from build123d import *

# Parameters (mm, degrees)
SKIZZE1_R                       = 18.5
LINEAR_AUSTRAGEN1_DEPTH         = 1.8
SKIZZE2_R                       = 23.4
SKIZZE2_R_2                     = 18.5
LINEAR_AUSTRAGEN2_DEPTH         = 1
SKIZZE3_R                       = 1
SCHNITT_LINEAR_AUSTRAGEN1_DEPTH = 34.832857329
CHAMFER1_SIZE                   = 1.4
SKETCH1_R                       = 5
CUT_EXTRUDE1_DEPTH              = 10


with BuildPart() as part:
    # Skizze1 → Linear austragen1 (new body)
    with BuildSketch(Plane.XY):
        with BuildLine():
            ThreePointArc((-22.806936421, 5.234849671), (-23.4, 0), (-22.806936421, -5.234849671))
            ThreePointArc((-22.806936421, -5.234849671), (-22.254722481, -7.230997668), (-21.528166589, -9.170498531))
            ThreePointArc((-21.528166589, -9.170498531), (-21.322328126, -10.083900652), (-21.453393631, -11.010990043))
            ThreePointArc((-21.453393631, -11.010990043), (-21.560643818, -12.043510102), (-21.221833257, -13.024737741))
            ThreePointArc((-21.221833257, -13.024737741), (-20.14452316, -14.635852782), (-18.94516883, -16.158297497))
            ThreePointArc((-18.94516883, -16.158297497), (-18.116664111, -16.783741505), (-17.10153705, -17.000806761))
            ThreePointArc((-17.10153705, -17.000806761), (-16.179321175, -17.162642436), (-15.37423172, -17.640663225))
            ThreePointArc((-15.37423172, -17.640663225), (-13.754174904, -18.930997668), (-12.026368835, -20.073027989))
            ThreePointArc((-12.026368835, -20.073027989), (-11.322957725, -20.690997014), (-10.884062474, -21.518066457))
            ThreePointArc((-10.884062474, -21.518066457), (-10.363929634, -22.416432811), (-9.513074997, -23.011114795))
            ThreePointArc((-9.513074997, -23.011114795), (-7.69452316, -23.681307256), (-5.829354574, -24.208028116))
            ThreePointArc((-5.829354574, -24.208028116), (-4.791453413, -24.227040092), (-3.842610612, -23.805972857))
            ThreePointArc((-3.842610612, -23.805972857), (-3.001397674, -23.394835778), (-2.069093052, -23.308343012))
            ThreePointArc((-2.069093052, -23.308343012), (0, -23.4), (2.069093052, -23.308343012))
            ThreePointArc((2.069093052, -23.308343012), (3.001397674, -23.394835778), (3.842610612, -23.805972857))
            ThreePointArc((3.842610612, -23.805972857), (4.791453413, -24.227040092), (5.829354574, -24.208028116))
            ThreePointArc((5.829354574, -24.208028116), (7.69452316, -23.681307256), (9.513074997, -23.011114795))
            ThreePointArc((9.513074997, -23.011114795), (10.363929634, -22.416432811), (10.884062474, -21.518066457))
            ThreePointArc((10.884062474, -21.518066457), (11.322957725, -20.690997014), (12.026368835, -20.073027989))
            ThreePointArc((12.026368835, -20.073027989), (13.754174904, -18.930997668), (15.37423172, -17.640663225))
            ThreePointArc((15.37423172, -17.640663225), (16.179321175, -17.162642436), (17.10153705, -17.000806761))
            ThreePointArc((17.10153705, -17.000806761), (18.116664111, -16.783741505), (18.94516883, -16.158297497))
            ThreePointArc((18.94516883, -16.158297497), (20.14452316, -14.635852782), (21.221833257, -13.024737741))
            ThreePointArc((21.221833257, -13.024737741), (21.560643818, -12.043510102), (21.453393631, -11.010990043))
            ThreePointArc((21.453393631, -11.010990043), (21.322328126, -10.083900652), (21.528166589, -9.170498531))
            ThreePointArc((21.528166589, -9.170498531), (22.254722481, -7.230997668), (22.806936421, -5.234849671))
            ThreePointArc((22.806936421, -5.234849671), (23.4, 0), (22.806936421, 5.234849671))
            ThreePointArc((22.806936421, 5.234849671), (22.254722481, 7.230997668), (21.528166589, 9.170498531))
            ThreePointArc((21.528166589, 9.170498531), (21.322328126, 10.083900652), (21.453393631, 11.010990043))
            ThreePointArc((21.453393631, 11.010990043), (21.560643818, 12.043510102), (21.221833257, 13.024737741))
            ThreePointArc((21.221833257, 13.024737741), (20.14452316, 14.635852782), (18.94516883, 16.158297497))
            ThreePointArc((18.94516883, 16.158297497), (18.116664111, 16.783741505), (17.10153705, 17.000806761))
            ThreePointArc((17.10153705, 17.000806761), (16.179321175, 17.162642436), (15.37423172, 17.640663225))
            ThreePointArc((15.37423172, 17.640663225), (13.754174904, 18.930997668), (12.026368835, 20.073027989))
            ThreePointArc((12.026368835, 20.073027989), (11.322957725, 20.690997014), (10.884062474, 21.518066457))
            ThreePointArc((10.884062474, 21.518066457), (10.363929634, 22.416432811), (9.513074997, 23.011114795))
            ThreePointArc((9.513074997, 23.011114795), (7.69452316, 23.681307256), (5.829354574, 24.208028116))
            ThreePointArc((5.829354574, 24.208028116), (4.791453413, 24.227040092), (3.842610612, 23.805972857))
            ThreePointArc((3.842610612, 23.805972857), (3.001397674, 23.394835778), (2.069093052, 23.308343012))
            ThreePointArc((2.069093052, 23.308343012), (0, 23.4), (-2.069093052, 23.308343012))
            ThreePointArc((-2.069093052, 23.308343012), (-3.001397674, 23.394835778), (-3.842610612, 23.805972857))
            ThreePointArc((-3.842610612, 23.805972857), (-4.791453413, 24.227040092), (-5.829354574, 24.208028116))
            ThreePointArc((-5.829354574, 24.208028116), (-7.69452316, 23.681307256), (-9.513074997, 23.011114795))
            ThreePointArc((-9.513074997, 23.011114795), (-10.363929634, 22.416432811), (-10.884062474, 21.518066457))
            ThreePointArc((-10.884062474, 21.518066457), (-11.322957725, 20.690997014), (-12.026368835, 20.073027989))
            ThreePointArc((-12.026368835, 20.073027989), (-13.754174904, 18.930997668), (-15.37423172, 17.640663225))
            ThreePointArc((-15.37423172, 17.640663225), (-16.179321175, 17.162642436), (-17.10153705, 17.000806761))
            ThreePointArc((-17.10153705, 17.000806761), (-18.116664111, 16.783741505), (-18.94516883, 16.158297497))
            ThreePointArc((-18.94516883, 16.158297497), (-20.14452316, 14.635852782), (-21.221833257, 13.024737741))
            ThreePointArc((-21.221833257, 13.024737741), (-21.560643818, 12.043510102), (-21.453393631, 11.010990043))
            ThreePointArc((-21.453393631, 11.010990043), (-21.322328126, 10.083900652), (-21.528166589, 9.170498531))
            ThreePointArc((-21.528166589, 9.170498531), (-22.254722481, 7.230997668), (-22.806936421, 5.234849671))
        make_face()
        Circle(SKIZZE1_R, mode=Mode.SUBTRACT)
    extrude(amount=LINEAR_AUSTRAGEN1_DEPTH)

    # Skizze2 → Linear austragen2 (add)
    with BuildSketch(Plane.XY.offset(1.8)):
        with Locations(Location((0, 0, 0), (0, 0, 156.927122734))):
            Circle(SKIZZE2_R)
        Circle(SKIZZE2_R_2, mode=Mode.SUBTRACT)
    extrude(amount=LINEAR_AUSTRAGEN2_DEPTH)

    # Skizze3 → Schnitt-Linear austragen1 (cut, through all)
    with BuildSketch(Plane.XY.offset(2.8)):
        with Locations((-6.643865379, 20.4477151)):
            Circle(SKIZZE3_R)
        with Locations((6.643865379, 20.4477151)):
            Circle(SKIZZE3_R)
        with Locations((17.393865379, 12.637382924)):
            Circle(SKIZZE3_R)
        with Locations((17.393865379, -12.637382924)):
            Circle(SKIZZE3_R)
        with Locations((6.643865379, -20.4477151)):
            Circle(SKIZZE3_R)
        with Locations((-6.643865379, -20.4477151)):
            Circle(SKIZZE3_R)
        with Locations((-17.393865379, -12.637382924)):
            Circle(SKIZZE3_R)
        with Locations((-17.393865379, 12.637382924)):
            Circle(SKIZZE3_R)
    extrude(amount=-SCHNITT_LINEAR_AUSTRAGEN1_DEPTH, mode=Mode.SUBTRACT)

    # Chamfer1
    chamfer1_edges = [part.edges().sort_by_distance(p)[0] for p in [
        (-7.643865379, 20.4477151, 0),
        (5.643865379, 20.4477151, 0),
        (16.393865379, 12.637382924, 0),
        (16.393865379, -12.637382924, 0),
        (5.643865379, -20.4477151, 0),
        (-7.643865379, -20.4477151, 0),
        (-18.393865379, -12.637382924, 0),
        (-18.393865379, 12.637382924, 0),
    ]]
    chamfer(chamfer1_edges, length=CHAMFER1_SIZE)

    # Sketch1 → Cut-Extrude1 (cut)
    with BuildSketch(Plane(origin=(0, 0, 0), x_dir=(-1, 0, 0), z_dir=(0, 0, -1))):
        with Locations((-25, 0)):
            Circle(SKETCH1_R)
        with Locations((25, 0)):
            Circle(SKETCH1_R)
    extrude(amount=-CUT_EXTRUDE1_DEPTH, mode=Mode.SUBTRACT)


solid = part.part
Can you work these out from the model? Positions are in its coordinate system, mm. Give positions to 0.01 mm unless a question says otherwise; leave off trailing zeros. Order: outer loops, then holes, each group sorted by start corner. A loop starts at its lowest first (then second) coordinate and runs counter-clockwise, first axis right, second up. Notation, with made-up numbers: M 27,18.5 L 73,18.5 A20 ccw 73,24.5 Z; hole C 22.5,14 d2. An arc over 180 degrees is marked long. Use a Markdown table: item, result. Add a question column.
Item 1: Suppose I cut it at C-C (z = 2.3). Count the separate pieces of the cut face and the enclosed holes in it, then the cut area to 3 significant figures.
Item 2: Suppose I cut it at D-D (y = 6). List the corners of the cut face in (x, z) for me.
Item 3: Will these pins go through, and if not, where does the flat tip stop? pin 1 (2.5 mm diameter, centred on x = 6.64, y = 20.45, fed in from -Z); pin 2 (1.3 mm diameter, centred on x = 9.5, y = -21.5, fed in from +Z).
Item 4: Suppose I cut it at A-A (x = 0). List the corners of the cut face in (y, z) for me, then the cut area to 3 significant figures.
Item 5: If I drill on L1, parallel to X at y = -20, z = 0.3; L2, parallel to Y at x = 6, z = 1.7; L3, parallel to X at y = -21, z = 0.9, over which ranges is the centre line in solid material (lowest first)? Write a range as [from, to].
Item 6: We'd pull the mould along X, two halves only. Please class faces 1 (the cylindrical face through (-7.67, 23.69, 0.89)), 2 (the cylindrical face through (21.562, 12.029, 0.887)), 3 (the cylindrical face through (-6.77, 21.44, 2.11)): +X half, -X half, draft (parallel to the pull), parting line (faces both ways), or undercut.
Item 7: Suppose I cut it at B-B (y = 0). List the corners of the cut face in (x, z) for me.
Answer sheet:
| question | item | result |
|---|---|---|
| 1 | separate pieces | 1 |
| 1 | enclosed holes | 9 |
| 1 | area | 576 mm² |
| 2 | outline | M -22.62,0 L -17.5,0 L -17.5,2.8 L -22.62,2.8 Z; M 17.5,0 L 22.62,0 L 22.62,2.8 L 17.5,2.8 Z |
| 3 | pin 1 | stops at z = 1.15 |
| 3 | pin 2 | stops at z = 2.8 |
| 4 | outline | M -23.4,0 L -18.5,0 L -18.5,2.8 L -23.4,2.8 Z; M 18.5,0 L 23.4,0 L 23.4,2.8 L 18.5,2.8 Z |
| 4 | area | 27.4 mm² |
| 5 | L1 | x = [-12.15, -8.7], [-4.59, 4.59], [8.7, 12.15] |
| 5 | L2 | y = [-24.17, -21.21], [-19.68, -17.5], [17.5, 19.68], [21.21, 24.17] |
| 5 | L3 | x = [-11.11, -8.04], [-5.25, 5.25], [8.04, 11.11] |
| 6 | face 1 | -X half |
| 6 | face 2 | +X half |
| 6 | face 3 | undercut |
| 7 | outline | M -20,0 L -18.5,0 L -18.5,2.8 L -20,2.8 Z; M 18.5,0 L 20,0 L 20,2.8 L 18.5,2.8 Z |
